Build history of the part. All positions in model axes, mm. A direction names the side the tool comes from. Coordinates: 2 decimals unless noted, no trailing zeros. Loops run counter-clockwise (first coordinate to the right, second up) from the corner with the lowest first, then second, coordinate; pieces in that order, holes last.
Item 1: Mould opens along X. For faces 1 (the face through (34, 24, 4)), 2 (the face through (40.533, 31.455, 1.972)), 3 (the face through (31.107, 25.785, 2.028)), 4 (the face through (54.45, 20.975, 1.972)) say: released by +X, released by -X, zero draft, split by the parting line, or undercut.
Item 2: Cut at D-D (x = 21.5). List the corners of the cut face in (y, z).
Item 3: Cut at A-A (x = 48). List the corners of the cut face in (y, z).
Item 4: Cut at C-C (x = 40). List the corners of the cut face in (y, z), and give its area (3 significant figures).
Item 5: Cut at B-B (z = 1.6). List the corners of the cut face in (x, y) (3 decimals).
Item 6: Drill centre lines: line 1 along X through (y, z) = (24.25, 2.85); line 2 along X through (y, z) = (23.25, 3.2); line 3 along X through (y, z) = (22.75, 3.8). Where is each one in solid material? Low to high.
Item 7: 3-axis set-ups, long thin cutter, end or side, ignore diameter. For faces 5 (the face through (31, 17.899, 2)), 6 (the face through (21, 27.899, 2)): which of +Z, -Z, +X, -X, +Y, -Y reach the whole face in a straight line?
from build123d import *

# Parameters (mm, degrees)
SKETCH_1_R          = 1.65
EXTRUDE_1_DEPTH     = 4
SKETCH_2_W          = 37.773502691
SKETCH_2_H          = 11.965737329
CUT_EXTRUDE_1_DEPTH = 10
SKETCH_4_R          = 1.65
CUT_EXTRUDE_3_DEPTH = 10
CUT_EXTRUDE_2_DEPTH = 10
FILLET_1_R          = 20
SKETCH_5_R          = 1.525
CUT_EXTRUDE_4_DEPTH = 12


with BuildPart() as part:
    # 草图1 → 凸台-拉伸1 (new body)
    with BuildSketch(Plane.XY):
        with BuildLine():
            Line((13.169415516, 42.898917412), (45.169415516, 42.898917412))
            Line((45.169415516, 42.898917412), (54.407019823, 26.898917412))
            ThreePointArc((54.407019823, 26.898917412), (54.407019823, 20.898917412), (49.2108674, 17.898917412))
            Line((49.2108674, 17.898917412), (25.169415516, 17.898917412))
            Line((25.169415516, 17.898917412), (13.169415516, 17.898917412))
            Line((13.169415516, 17.898917412), (13.169415516, 42.898917412))
        make_face()
        with Locations((49.2108674, 23.898917412)):
            Circle(SKETCH_1_R, mode=Mode.SUBTRACT)
    extrude(amount=EXTRUDE_1_DEPTH)

    # 草图2 → 切除-拉伸1 (cut)
    with BuildSketch(Plane.XY.offset(4)):
        with Locations((32.056166862, 38.881786077)):
            Rectangle(SKETCH_2_W, SKETCH_2_H)
    extrude(amount=-CUT_EXTRUDE_1_DEPTH, mode=Mode.SUBTRACT)

    # 草图4 → 切除-拉伸3 (cut)
    with BuildSketch(Plane.XY.offset(4)):
        with Locations((19.287444113, 22.898917412)):
            Circle(SKETCH_4_R)
        with Locations((39.287444113, 26.898917412)):
            Circle(SKETCH_4_R)
    extrude(amount=-CUT_EXTRUDE_3_DEPTH, mode=Mode.SUBTRACT)

    # 草图3 → 切除-拉伸2 (cut)
    with BuildSketch(Plane(origin=(0, 0, 0), x_dir=(-1, 0, 0), z_dir=(0, 0, -1))):
        with BuildLine():
            Line((-13.169415516, 27.898917412), (-33.118062206, 27.898917412))
            ThreePointArc((-33.118062206, 27.898917412), (-38.100309763, 30.092049708), (-42.764440301, 32.898917412))
            Line((-42.764440301, 32.898917412), (-13.169415516, 32.898917412))
            Line((-13.169415516, 32.898917412), (-13.169415516, 27.898917412))
        make_face()
    extrude(amount=-CUT_EXTRUDE_2_DEPTH, mode=Mode.SUBTRACT)

    # 圆角1
    fillet_1_edges = [part.edges().sort_by_distance(p)[0] for p in [
        (33.118062206, 27.898917412, 2),
    ]]
    fillet(fillet_1_edges, radius=FILLET_1_R)

    # 草图5 → 切除-拉伸4 (cut)
    with BuildSketch(Plane.XY.offset(4)):
        with Locations((30.287444113, 24.499597572)):
            Circle(SKETCH_5_R)
        with Locations((45.287444113, 30.764768776)):
            Circle(SKETCH_5_R)
    extrude(amount=-CUT_EXTRUDE_4_DEPTH, mode=Mode.SUBTRACT)


solid = part.part
Filled sheet:
1. face 1: zero draft
1. face 2: released by -X
1. face 3: undercut
1. face 4: released by +X
2. outline: (17.9, 0) - (27.9, 0) - (27.9, 4) - (17.9, 4) - close
3. outline: (17.9, 0) - (22.78, 0) - (22.78, 4) - (17.9, 4) - close; (25.02, 0) - (32.9, 0) - (32.9, 4) - (25.02, 4) - close
4. outline: (17.9, 0) - (25.41, 0) - (25.41, 4) - (17.9, 4) - close; (28.39, 0) - (31.14, 0) - (31.14, 4) - (28.39, 4) - close
4. area: 41.1 mm2
5. outline: (13.169, 17.899) - (49.211, 17.899) arc R6 ccw to (54.407, 26.899) - (50.943, 32.899) - (42.764, 32.899) arc R42.866 cw to (38.282, 30.187) arc R20 cw to (28.993, 27.899) - (13.169, 27.899) - close; hole circle Ø3.3 at (19.287, 22.899); hole circle Ø3.05 at (30.287, 24.5); hole circle Ø3.3 at (39.287, 26.899); hole circle Ø3.05 at (45.287, 30.765); hole circle Ø3.3 at (49.211, 23.899)
6. line 1: x = 13.17 to 18.34, 20.23 to 28.78, 31.79 to 47.6, 50.82 to 55.2
6. line 2: x = 13.17 to 17.68, 20.9 to 29.41, 31.16 to 47.69, 50.73 to 55.18
6. line 3: x = 13.17 to 17.64, 20.93 to 48.03, 50.4 to 55.1
7. face 5: +Z, -Z, +X, -X, -Y
7. face 6: +Z, -Z, -X, +Y
